from build123d import *

# Parameters (mm, degrees)
SKETCH_1_W          = 140
SKETCH_1_H          = 140
EXTRUDE_1_DEPTH     = 5
SKETCH_2_R          = 4
CUT_EXTRUDE_1_DEPTH = 5
SKETCH_3_R          = 7.5
EXTRUDE_2_DEPTH     = 16
EXTRUDE_3_DEPTH     = 131
SKETCH_5_R          = 40
EXTRUDE_4_DEPTH     = 20


with BuildPart() as part:
    # 草图1 → 凸台-拉伸1 (new body)
    with BuildSketch(Plane(origin=(0, 0, 0), x_dir=(1, 0, 0), z_dir=(0, 1, 0))):
        Rectangle(SKETCH_1_W, SKETCH_1_H)
    extrude(amount=EXTRUDE_1_DEPTH)

    # 草图2 → 切除-拉伸1 (cut)
    with BuildSketch(Plane(origin=(0, 5, 0), x_dir=(1, 0, 0), z_dir=(0, 1, 0))):
        with Locations(Location((-54, 54, 0), (0, 0, 270))):
            Circle(SKETCH_2_R)
        with Locations(Location((54, 54, 0), (0, 0, 270))):
            Circle(SKETCH_2_R)
        with Locations(Location((54, -54, 0), (0, 0, 270))):
            Circle(SKETCH_2_R)
        with Locations(Location((-54, -54, 0), (0, 0, 270))):
            Circle(SKETCH_2_R)
    extrude(amount=-CUT_EXTRUDE_1_DEPTH, mode=Mode.SUBTRACT)

    # 草图3 → 凸台-拉伸2 (add)
    with BuildSketch(Plane(origin=(0, 5, 0), x_dir=(1, 0, 0), z_dir=(0, 1, 0))):
        with Locations(Location((0, 0, 0), (0, 0, 270))):
            Circle(SKETCH_3_R)
    extrude(amount=-EXTRUDE_2_DEPTH)

    # 草图4 → 凸台-拉伸3 (add)
    with BuildSketch(Plane(origin=(0, 5, 0), x_dir=(1, 0, 0), z_dir=(0, 1, 0))):
        with BuildLine():
            Line((-43.0341439, -60), (43.0341439, -60))
            ThreePointArc((43.0341439, -60), (45.161165235, -45.161165235), (60, -43.0341439))
            Line((60, -43.0341439), (60, 43.0341439))
            ThreePointArc((60, 43.0341439), (45.161165235, 45.161165235), (43.0341439, 60))
            Line((43.0341439, 60), (-43.0341439, 60))
            ThreePointArc((-43.0341439, 60), (-45.161165235, 45.161165235), (-60, 43.0341439))
            Line((-60, 43.0341439), (-60, -43.0341439))
            ThreePointArc((-60, -43.0341439), (-45.161165235, -45.161165235), (-43.0341439, -60))
        make_face()
    extrude(amount=EXTRUDE_3_DEPTH)

    # 草图5 → 凸台-拉伸4 (add)
    with BuildSketch(Plane(origin=(0, 136, 0), x_dir=(1, 0, 0), z_dir=(0, 1, 0))):
        with Locations(Location((0, 0, 0), (0, 0, 270))):
            Circle(SKETCH_5_R)
    extrude(amount=EXTRUDE_4_DEPTH)


solid = part.part
Here's how the part is built. I have some questions about the finished solid (model axes, mm). A direction names the side the tool comes from. Coordinates: 2 decimals unless noted, no trailing zeros. Order: outer loops, then holes, each group sorted by start corner. A loop starts at its lowest first (then second) coordinate and runs counter-clockwise, first axis right, second up. Notation, with made-up numbers: M 20.25,86.25 L 43.25,86.25 A14 cw 43.25,112.25 Z; hole C 41.25,79.25 d10. An arc over 180 degrees is marked long. Answer as CSV lines item,"result". Start each with the question number.
1. We'd pull the mould along X, two halves only. Please class faces 1 (the flat face through (-70, 2, 1)), 2 (the flat face through (-1, 2, 70)), 3 (the cylindrical face through (45.322, 69.583, -45.003)): released by +X, released by -X, zero draft, split by the parting line, or undercut.
2. For pin 1 (12 mm diameter, centred on x = -10, y = 74.5, fed in from +Z); pin 2 (8 mm diameter, centred on y = 22, z = -24, fed in from +X); pin 3 (1 mm diameter, centred on x = 24, y = 130.5, fed in from -Z); pin 4 (7 mm diameter, centred on x = -54, z = 54, fed in from +Y), each with a flat end and sliding along its axis, tell me the tip position at first contact or that it passes through.
3. I need wall thicknesses on line 1 (X direction, y = 2.6, z = -54); line 2 (Y direction, x = -56, z = 36); line 3 (Z direction, x = -13, y = 24.5). Which ranges of each line are inside material? Lowest first, please. Write a range as [from, to].
4. I want a section at B-B, the plane x = 0. Write out the boundary of the cut face in (y, z), and give its area (3 significant figures).
5. I want a section at C-C, the plane y = 54. Write out the boundary of the cut face in (x, z).
6. I want a section at A-A, the plane z = -54. Write out the boundary of the cut face in (x, y), and give its area (3 significant figures).
7. I want a section at D-D, the plane x = 54. Write out the boundary of the cut face in (y, z).
8. On a 3-axis mill with a long thin cutter (end or side, diameter ignored), from which of +Z, -Z, +X, -X, +Y, -Y can I reach the whole of each face in a straight line? I mean faces 4 (the cylindrical face through (0.33, -5.423, -7.493)), 5 (the flat face through (-1, 70, 60)), 6 (the flat face through (-60, 70, -1)), 7 (the flat face through (-1, 136, -41)). Say none if no direction works.
Recorded:
1,face 1,"released by -X"
1,face 2,"zero draft"
1,face 3,"undercut"
2,pin 1,"stops at z = 60"
2,pin 2,"stops at x = 60"
2,pin 3,"stops at z = -60"
2,pin 4,"passes through"
3,line 1,"x = [-70, -58], [-50, 50], [58, 70]"
3,line 2,"y = [0, 136]"
3,line 3,"z = [-60, 60]"
4,outline,"M -11,-7.5 L 0,-7.5 L 0,-70 L 5,-70 L 5,-60 L 136,-60 L 136,-40 L 156,-40 L 156,40 L 136,40 L 136,60 L 5,60 L 5,70 L 0,70 L 0,7.5 L -11,7.5 Z"
4,area,"18,200 mm2"
5,outline,"M -60,-43.03 A12.5 cw -43.03,-60 L 43.03,-60 A12.5 cw 60,-43.03 L 60,43.03 A12.5 cw 43.03,60 L -43.03,60 A12.5 cw -60,43.03 Z"
6,outline,"M -70,0 L -58,0 L -58,5 L -70,5 Z; M -50,0 L 50,0 L 50,5 L 41.5,5 L 41.5,136 L -41.5,136 L -41.5,5 L -50,5 Z; M 58,0 L 70,0 L 70,5 L 58,5 Z"
6,area,"11,500 mm2"
7,outline,"M 0,-70 L 5,-70 L 5,-58 L 0,-58 Z; M 0,-50 L 5,-50 L 5,-41.5 L 136,-41.5 L 136,41.5 L 5,41.5 L 5,50 L 0,50 Z; M 0,58 L 5,58 L 5,70 L 0,70 Z"
8,face 4,"-Y"
8,face 5,"+Z, +X, -X, +Y"
8,face 6,"+Z, -Z, -X, +Y"
8,face 7,"+Y"
